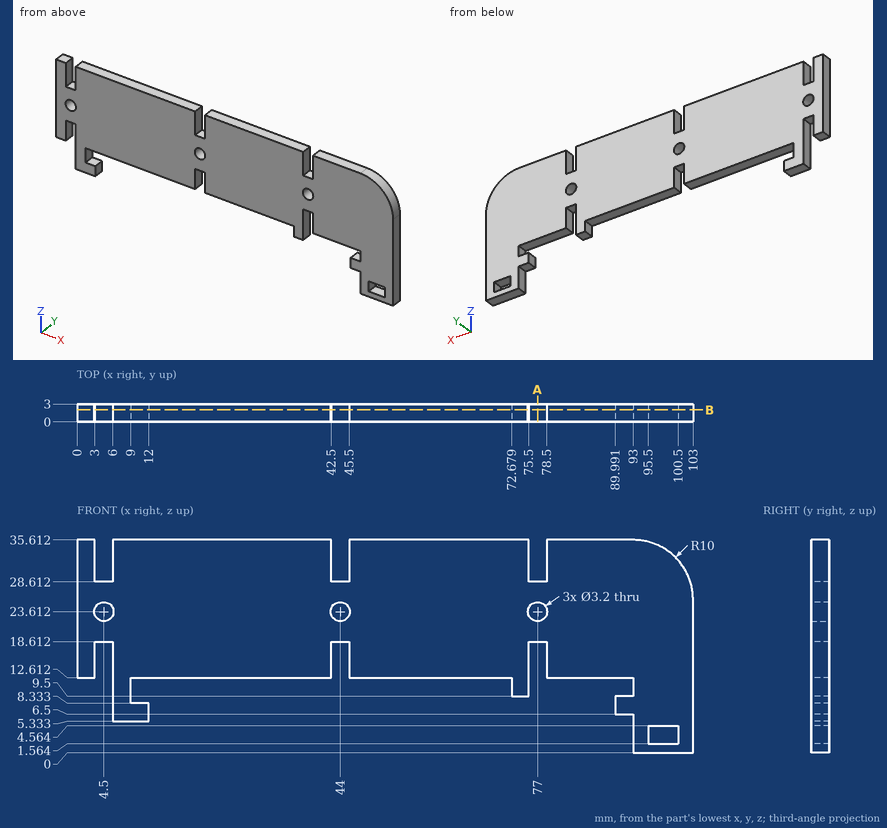
For this review, use the dimensioned drawing (mm, ordinates from the lowest corner) and the shaded views. Give positions to 0.01 mm unless a question says otherwise; leave off trailing zeros. Order: outer loops, then holes, each group sorted by start corner. A loop starts at its lowest first (then second) coordinate and runs counter-clockwise, first axis right, second up. Notation, with made-up numbers: (77.25, 1.5) -> (113.25, 1.5) arc R36 ccw to (113.25, 37.5) -> close; hole circle Ø3 at (-36.5, -24). An arc over 180 degrees is marked (long way). Write item = value, one per line. Start each with the question number.
(1) Take a section at A-A (x = 77). Write out the cut boundary in (y, z), plus the area to 3 significant figures.
(2) For L1, parallel to X at y = 1.6, z = 10.5; L2, parallel to X at y = 1.2, z = 16; L3, parallel to X at y = 1, z = 25 (1 decimal), list the stretches that pass through material, from the lowest coordinate up. Write a range as from..to.
(3) For pin 1 Ø4 at (x, z) = (44, 23.61) entering from -Y; pin 2 Ø1.5 at (y, z) = (2.5, 30.5) entering from +X; pin 3 Ø0.9 at (y, z) = (2, 33.5) entering from +X (1 decimal); pin 4 Ø0.9 at (y, z) = (1, 31.5) entering from +X, all flat-tipped, find the tip position at first contact; note any pin that passes through.
(4) Take a section at B-B (y = 2). State how many separate pieces and enclosed holes the cut face has, plus the area to 3 significant figures.
Returned:
q1.outline = (0, 18.61) -> (3, 18.61) -> (3, 22.01) -> (0, 22.01) -> close; (0, 25.21) -> (3, 25.21) -> (3, 28.61) -> (0, 28.61) -> close
q1.area = 20.4 mm²
q2.L1 = 6..9, 72.68..75.5, 93..103
q2.L2 = 0..3, 6..42.5, 45.5..75.5, 78.5..103
q2.L3 = 0..3.7, 5.3..43.2, 44.8..76.2, 77.8..103
q3.pin_1 = 0
q3.pin_2 = 102.1
q3.pin_3 = 99.7
q3.pin_4 = 101.39
q4.separate_pieces = 1
q4.enclosed_holes = 4
q4.area = 2,370 mm²
